The listing builds one solid part. Answer for the finished solid, in the listing's coordinates (mm). A direction names the side the tool comes from. Coordinates: 2 decimals unless noted, no trailing zeros. Loops run counter-clockwise (first coordinate to the right, second up) from the corner with the lowest first, then second, coordinate; pieces in that order, holes last. Notation, with made-up numbers: M 22.25,12.25 L 64.25,12.25 A21 ccw 64.25,22.25 Z; hole C 75,73 d10. An arc over 180 degrees is marked long. Return JSON: item names as keys, results as strings. Group by question number.
1. The mould has two halves that part along X. Classify faces 1 (the face through (-11, -4, 3)), 2 (the face through (6.2, -14, 3.5)), 3 (the face through (-15.8, -10, 3)): pulls with the +X half, pulls with the -X half, needs draft (parallel to the pull), parting line crosses it, or undercut.
2. Section C-C (x = 0) is taken. Write down the section's boundary in (y, z).
3. Straight lines are drawn through the part: L1, parallel to X at y = 0, z = 2.5; L2, parallel to X at y = -7.25, z = 6; L3, parallel to Y at x = -3.5, z = 5. For each, find the intervals that lie inside material, in ascending order. Write a range as from..to.
4. Section B-B (z = 3.5) is taken. Write down the section's boundary in (x, y).
5. Section D-D (x = -7.25) is taken. Write down the section's boundary in (y, z), then the cut area to 3 significant figures.
6. Section A-A (y = -10.5) is taken. Write down the section's boundary in (x, z).
7. Given P1, Ø1.1, axis at x = -13.5, z = 2.5, coming from the +Y side; P2, Ø4, axis at x = 1, z = 3, coming from the -Y side; P3, Ø3, axis at y = 4.5, z = 3.5, coming from the -X side, each flat-ended and moving along its own axis, determine where each tip first touches the part or whether it passes through.
8. Which of the six approach directions +Z, -Z, +X, -X, +Y, -Y give full straight-line access (tool end or side, diameter ignored) to faces 4 (the face through (-13.3, -13, 3.5)), 5 (the face through (-6.8, 1, 3)), 6 (the face through (-1, -4.4, 7)), 7 (the face through (-2.8, 5, 3))?
```python
from build123d import *

# Parameters (mm, degrees)
PAD_DEPTH = 7


with BuildPart() as part:
    # Sketch → Pad (new body)
    with BuildSketch(Plane.XY):
        with BuildLine():
            ThreePointArc((-2.8, 3.130495), (-1.714643, -3.834058), (4.2, 0))
            Line((4.2, 6), (4.2, 0))
            Line((4.2, 6), (8.2, 6))
            Line((8.2, 6), (8.2, -15))
            Line((8.2, -15), (7.2, -15))
            Line((7.2, -15), (5.2, -13))
            Line((5.2, -13), (6.2, -13))
            Line((6.2, -13), (6.2, -6))
            Line((6.2, -6), (-13.8, -6))
            Line((-13.8, -6), (-13.8, -13))
            Line((-13.8, -13), (-12.8, -13))
            Line((-12.8, -13), (-14.8, -15))
            Line((-14.8, -15), (-15.8, -15))
            Line((-15.8, -15), (-15.8, -4))
            Line((-15.8, -4), (-6.8, -4))
            Line((-6.8, -4), (-6.8, 6))
            Line((-6.8, 6), (-2.8, 6))
            Line((-2.8, 6), (-2.8, 3.130495))
        make_face()
    extrude(amount=PAD_DEPTH)


solid = part.part
```
Worked out:
{
 "1": {"face 1": "needs draft", "face 2": "undercut", "face 3": "pulls with the -X half"},
 "2": {"outline": "M -6,0 L -4.2,0 L -4.2,7 L -6,7 Z"},
 "3": {"L1": "-6.8..-4.2, 4.2..8.2", "L2": "-15.8..-13.8, 6.2..8.2", "L3": "-6..-2.32, 2.32..6"},
 "4": {"outline": "M -15.8,-15 L -14.8,-15 L -12.8,-13 L -13.8,-13 L -13.8,-6 L 6.2,-6 L 6.2,-13 L 5.2,-13 L 7.2,-15 L 8.2,-15 L 8.2,6 L 4.2,6 L 4.2,0 A4.2 cw long -2.8,3.13 L -2.8,6 L -6.8,6 L -6.8,-4 L -15.8,-4 Z"},
 "5": {"outline": "M -6,0 L -4,0 L -4,7 L -6,7 Z", "area": "14.0 mm^2"},
 "6": {"outline": "M -15.8,0 L -13.8,0 L -13.8,7 L -15.8,7 Z; M 6.2,0 L 8.2,0 L 8.2,7 L 6.2,7 Z"},
 "7": {"P1": "y = -4", "P2": "y = -6", "P3": "x = -6.8"},
 "8": {"face 4": "+Z, -Z", "face 5": "+Z, -Z, -X, +Y", "face 6": "+Z, +X, -X, +Y, -Y", "face 7": "+Z, -Z, +Y"}
}
